Autodesk Inventor part; units mm, degrees
ref_plane "YZ Plane" through (0, 0, 0) normal (1, 0, 0) x (0, 1, 0)
ref_plane "XZ Plane" through (0, 0, 0) normal (0, 1, 0) x (-1, 0, 0)
ref_plane "XY Plane" through (0, 0, 0) normal (0, 0, 1) x (1, 0, 0)
sketch "Sketch1" plane through (0, 0, 0) normal (0, 0, 1) x (1, 0, 0)
  line L0 (-9.5, 12.3) -> (9.5, 12.3)
  line L1 (9.5, 12.3) -> (9.5, 0)
  line L2 (9.5, 0) -> (-9.5, 0)
  line L3 (-9.5, 0) -> (-9.5, 12.3)
  line L4 (-9.5, 12.3) -> (9.5, 0) construction
  line L5 (9.5, 12.3) -> (-9.5, 0) construction
  point P0 (0, 0)
  point P1 (0, 6.15)
  dimension "d0" = 12.3
  dimension "d1" = 19
  dimension "d2" = 0
  dimension "d3" = 12.3
extrude "Extrusion1" add sketch "Sketch1" along normal mid plane 5
sketch "Sketch2" plane through (0, 0, 0) normal (0, 0, 1) x (1, 0, 0)
  line L0 (-7.15, 1) -> (-7.15, -5.5)
  line L1 (-6.15, -6.5) -> (-2, -6.5)
  line L2 (-2, -6.5) -> (-2, -1)
  line L3 (-2, -1) -> (-3, -1)
  line L4 (-3, -1) -> (-3, 1)
  line L5 (-3, 1) -> (-7.15, 1)
  line L6 (-9.5, 0) -> (9.5, 0)
  line L7 (0, 0) -> (0, 7.1725) construction
  line L8 (-7.15, -5.5) -> (-6.15, -6.5)
  line L9 (7.15, 1) -> (7.15, -5.5)
  line L10 (6.15, -6.5) -> (2, -6.5)
  line L11 (2, -6.5) -> (2, -1)
  line L12 (2, -1) -> (3, -1)
  line L13 (3, -1) -> (3, 1)
  line L14 (3, 1) -> (7.15, 1)
  line L15 (7.15, -5.5) -> (6.15, -6.5)
  point P0 (-7.15, -6.5)
  point P1 (7.15, -6.5)
  dimension "d6" = 6.5
  dimension "d7" = 2
  dimension "d8" = 7.15
  dimension "d9" = 1
  dimension "d10" = 1
  dimension "d11" = 1
  dimension "d12" = 1
  dimension "d13" = 1
extrude "Extrusion2" add sketch "Sketch2" along normal mid plane 0.64
sketch "Sketch3" plane through (9.5, 0, 2.5) normal (1, 0, 0) x (0, 0, -1)
  line L0 (0, 12.3) -> (5, 12.3)
  line L1 (0, 0) -> (0, 12.3)
  line L2 (0, 0) -> (5, 0)
  line L3 (5, 12.3) -> (5, 0)
  line L4 (-1.5, 10.3) -> (0.75, 10.3)
  line L5 (0.75, 10.3) -> (1.5, 0)
  line L6 (-1.5, 10.3) -> (-1.5, -2)
  line L7 (-1.5, -2) -> (1.5, -2)
  line L8 (1.5, -2) -> (1.5, 0)
  line L9 (2.5, 0) -> (2.5, 10.8693) construction
  line L10 (6.5, 10.3) -> (4.25, 10.3)
  line L11 (4.25, 10.3) -> (3.5, 0)
  line L12 (6.5, 10.3) -> (6.5, -2)
  line L13 (6.5, -2) -> (3.5, -2)
  line L14 (3.5, 0) -> (3.5, -2)
  dimension "d16" = 2
  dimension "d17" = 0.75
  dimension "d18" = 1.5
  dimension "d19" = 2
  dimension "d20" = 1.5
extrude "Extrusion3" cut sketch "Sketch3" against normal through all contours L4 L5 L2 L1 | L1 L2 L8 L7 L6 L4 | L10 L12 L13 L14 L2 L3 | L3 L2 L11 L10
properties part number "ATCFuse"
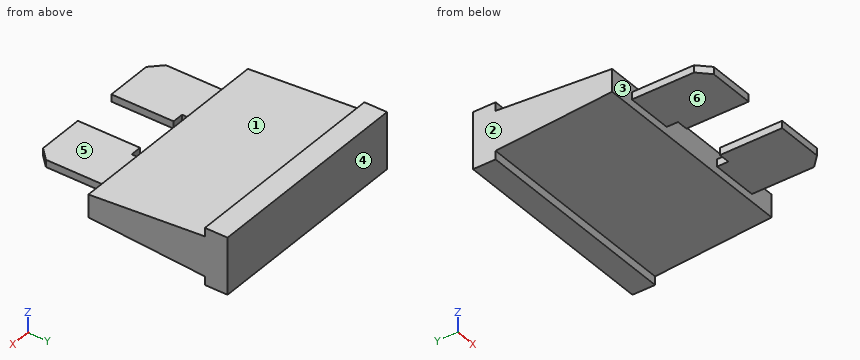
Geometry: final body of the model. Coordinates: model frame, mm. Face numbers are marked on the shaded views. A direction names the side the tool comes from. Coordinates: 2 decimals unless noted, no trailing zeros. Order: outer loops, then holes, each group sorted by start corner. A loop starts at its lowest first (then second) coordinate and runs counter-clockwise, first axis right, second up.
(1) Access query for the marked faces 4, 5 and 6. Directions: +Z, -Z, +X, -X, +Y, -Y. A direction counts if a zero-diameter tool reaches every point of the face in a straight line with its end or side. Return the directions, or none.
(2) First-contact query: pin 1 (4 mm diameter, centred on x = -3.5, y = -2.5, fed in from -Z); pin 2 (4 mm diameter, centred on x = -4, y = -3, fed in from +Z); pin 3 (0.5 mm diameter, centred on y = -2, z = 0, fed in from -X). Flat tips, straight axial feed; report the tip coordinate or a pass-through.
(3) Draft query along X for the marked faces 1, 2 and 3. Return one class per face: pulls with the +X half, pulls with the -X half, needs draft (parallel to the pull), parting line crosses it, or undercut.
(4) Material intervals for probe 1 along Y at (x, z) = (-6, -0.7); probe 2 along Y at (x, z) = (3, 2.1); probe 3 along Z at (x, y) = (2.75, 3), sorted ascending.
(5) Section query D-D (y = 2.5). Return the cut outline in (x, z).
(6) Section query C-C (z = -0.1). Return the cut outline in (x, y).
(7) Section query A-A (x = 2.5). Return the cut outline in (y, z).
(8) Section query B-B (x = 5). Return the cut outline in (y, z), plus the area to 3 significant figures.
Solution:
1. face 4: +Z, -Z, +X, -X, +Y
1. face 5: +Z, +X, -X, -Y
1. face 6: -Z, +X, -X, -Y
2. pin 1: stops at z = -0.32
2. pin 2: stops at z = 0.32
2. pin 3: stops at x = -7.15
3. face 1: needs draft
3. face 2: pulls with the -X half
3. face 3: undercut
4. probe 1: y = 0 to 12.3
4. probe 2: y = 10.3 to 12.3
4. probe 3: z = -1.22 to 1.22
5. outline: (-9.5, -1.18) - (9.5, -1.18) - (9.5, 1.18) - (-9.5, 1.18) - close
6. outline: (-9.5, 0) - (-7.15, 0) - (-7.15, -5.5) - (-6.15, -6.5) - (-2, -6.5) - (-2, -1) - (-3, -1) - (-3, 0) - (3, 0) - (3, -1) - (2, -1) - (2, -6.5) - (6.15, -6.5) - (7.15, -5.5) - (7.15, 0) - (9.5, 0) - (9.5, 12.3) - (-9.5, 12.3) - close
7. outline: (-6.5, -0.32) - (-1, -0.32) - (-1, 0.32) - (-6.5, 0.32) - close; (0, -1) - (10.3, -1.75) - (10.3, -2.5) - (12.3, -2.5) - (12.3, 2.5) - (10.3, 2.5) - (10.3, 1.75) - (0, 1) - close
8. outline: (-6.5, -0.32) - (0, -0.32) - (0, -1) - (10.3, -1.75) - (10.3, -2.5) - (12.3, -2.5) - (12.3, 2.5) - (10.3, 2.5) - (10.3, 1.75) - (0, 1) - (0, 0.32) - (-6.5, 0.32) - close
8. area: 42.5 mm2
